CAD build for the part. Positions are in the model's coordinates, mm. Face numbers are marked on the shaded views. Round coordinates to 2 decimals unless told otherwise and drop trailing zeros. Order: outer loops, then holes, each group sorted by start corner. A loop starts at its lowest first (then second) coordinate and runs counter-clockwise, first axis right, second up. Notation, with made-up numbers: (17.25, -3.75) -> (63.25, -3.75) arc R24 cw to (63.25, 19.25) -> close; hole circle Ø6 at (23, -14). An arc over 180 degrees is marked (long way). Return JSON: item names as keys, results as strings. Group by question number.
Q1. Cut at A-A (x = -8.5). Write the cut outline in (y, z).
Q2. Mould opens along Y. For the marked faces 1, 2 and 3 say: +Y half, -Y half, draft (parallel to the pull), parting line (faces both ways), or undercut.
Q3. Probe line 1 along Y through (x, z) = (-17, 465); line 2 along Y through (x, z) = (-18.05, 445.6); line 3 along Z through (x, y) = (17, 10). List the from-to ranges inside material, lowest first.
Q4. Cut at B-B (z = 109). Write the cut outline in (x, y).
from build123d import *

# Parameters (mm, degrees)
SKETCH1_W               = 38
SKETCH1_H               = 38
SKETCH1_W_2             = 32
SKETCH1_H_2             = 32
BOSS_EXTRUDE1_DEPTH     = 475.6
CUT_EXTRUDE2_DEPTH      = 478.493832421
CUT_EXTRUDE2_DEPTH_BACK = 478.493832421
SKETCH3_R               = 2.5


with BuildPart() as part:
    # Sketch1 → Boss-Extrude1 (new body)
    with BuildSketch(Plane.XY):
        Rectangle(SKETCH1_W, SKETCH1_H)
        Rectangle(SKETCH1_W_2, SKETCH1_H_2, mode=Mode.SUBTRACT)
    extrude(amount=BOSS_EXTRUDE1_DEPTH)

    # Sketch3 → Cut-Extrude2 (cut, two sides: drawn at the far end of the back side and taken through both)
    with BuildSketch(Plane(origin=(19, 0, 0), x_dir=(0, 0, -1), z_dir=(1, 0, 0)).offset(-CUT_EXTRUDE2_DEPTH_BACK)):
        with Locations(Location((-465.6, 10, 0), (0, 0, 270))):
            Circle(SKETCH3_R)
        with Locations(Location((-445.6, 10, 0), (0, 0, 270))):
            Circle(SKETCH3_R)
        with Locations(Location((-445.6, -10, 0), (0, 0, 270))):
            Circle(SKETCH3_R)
        with Locations(Location((-465.6, -10, 0), (0, 0, 270))):
            Circle(SKETCH3_R)
    extrude(amount=CUT_EXTRUDE2_DEPTH + CUT_EXTRUDE2_DEPTH_BACK, mode=Mode.SUBTRACT)


solid = part.part
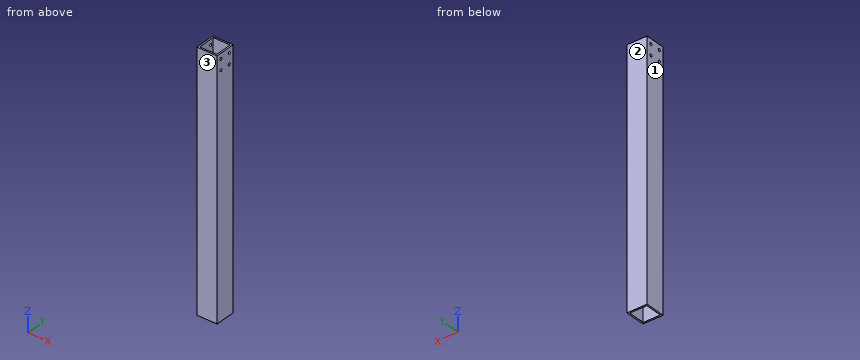
Solution:
{
 "1": {"outline": "(-19, 0) -> (-16, 0) -> (-16, 475.6) -> (-19, 475.6) -> close; (16, 0) -> (19, 0) -> (19, 475.6) -> (16, 475.6) -> close"},
 "2": {"face 1": "draft", "face 2": "+Y half", "face 3": "-Y half"},
 "3": {"line 1": "y = -19 to -12.43, -7.57 to 7.57, 12.43 to 19", "line 2": "y = -19 to -12.5, -7.5 to 7.5, 12.5 to 19", "line 3": "z = 0 to 443.1, 448.1 to 463.1, 468.1 to 475.6"},
 "4": {"outline": "(-19, -19) -> (19, -19) -> (19, 19) -> (-19, 19) -> close; hole (-16, -16) -> (16, -16) -> (16, 16) -> (-16, 16) -> close"}
}
